Answer from the drawing. Dimensions are ordinates in mm from the lowest x, y and z of the part. A direction names the side the tool comes from. Round coordinates to 2 decimals unless told otherwise and drop trailing zeros. Write each loop counter-clockwise with the first axis right and the second up, starting at its lowest first coordinate (ties: lowest second). Pieces come first, ordered by that corner, then holes. Notation, with made-up numbers: (80, -22.5) -> (120, -22.5) arc R35 ccw to (120, 10.5) -> close; hole circle Ø2 at (-39, -21). An arc over 180 degrees is marked (long way). Return JSON: item names as keys, results as strings. Group by question number.
(1) A cutting plane is placed at B-B on x = 17. Give the vertices of the cut face in (y, z), then the cut area to 3 significant figures.
(2) A cutting plane is placed at C-C on y = 2.5. Give the vertices of the cut face in (x, z), then the cut area to 3 significant figures.
(3) A cutting plane is placed at A-A on y = 18. Give the vertices of the cut face in (x, z), then the cut area to 3 significant figures.
(4) For the marked faces 4, 5 and 6, determine the directions among +Z, -Z, +X, -X, +Y, -Y from which every point of the face is accessible in a straight line to the end or side of a thin tool.
(5) Given pin 1 (3 mm diameter, centred on y = 8.5, z = 1.5, fed in from +X); pin 2 (2 mm diameter, centred on x = 12, y = 15, fed in from -Z); pin 3 (3 mm diameter, centred on y = 17, z = 2, fed in from -X); pin 4 (2 mm diameter, centred on x = 2, z = 3.5, fed in from +Y), each flat-ended and moving along its own axis, determine where each tip first touches the part or whether it passes through.
(6) A cutting plane is placed at D-D on z = 4.9. Give the vertices of the cut face in (x, y), then the cut area to 3 significant figures.
(7) The mould has two halves that part along Z. Classify the marked faces 1, 2 and 3: released by +Z, released by -Z, zero draft, split by the parting line, or undercut.
(8) Straight lines are drawn through the part: line 1 (X direction, y = 14.5, z = 4.8); line 2 (Y direction, x = 4.65, z = 3); line 3 (X direction, y = 3.25, z = 4.1). For each, find the intervals that lie inside material, in ascending order.
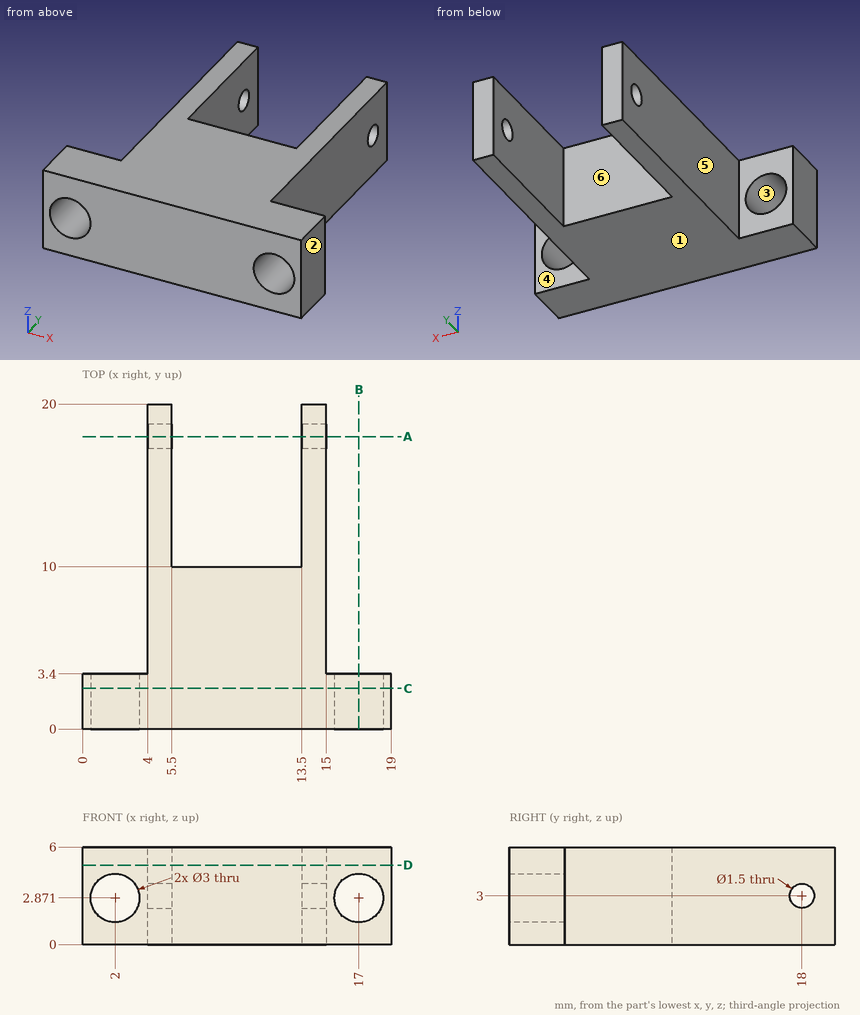
Checks:
{
 "1": {"outline": "(0, 0) -> (3.4, 0) -> (3.4, 1.37) -> (0, 1.37) -> close; (0, 4.37) -> (3.4, 4.37) -> (3.4, 6) -> (0, 6) -> close", "area": "10.2 mm^2"},
 "2": {"outline": "(0, 0) -> (19, 0) -> (19, 6) -> (0, 6) -> close; hole circle Ø3 at (2, 2.87); hole circle Ø3 at (17, 2.87)", "area": "99.9 mm^2"},
 "3": {"outline": "(4, 0) -> (5.5, 0) -> (5.5, 2.25) -> (4, 2.25) -> close; (4, 3.75) -> (5.5, 3.75) -> (5.5, 6) -> (4, 6) -> close; (13.5, 0) -> (15, 0) -> (15, 2.25) -> (13.5, 2.25) -> close; (13.5, 3.75) -> (15, 3.75) -> (15, 6) -> (13.5, 6) -> close", "area": "13.5 mm^2"},
 "4": {"face 4": "+Z, -Z, +X, +Y", "face 5": "+Z, -Z, -X, +Y", "face 6": "+Z, -Z, +Y"},
 "5": {"pin 1": "stops at x = 15", "pin 2": "passes through", "pin 3": "stops at x = 4", "pin 4": "stops at y = 3.4"},
 "6": {"outline": "(0, 0) -> (19, 0) -> (19, 3.4) -> (15, 3.4) -> (15, 20) -> (13.5, 20) -> (13.5, 10) -> (5.5, 10) -> (5.5, 20) -> (4, 20) -> (4, 3.4) -> (0, 3.4) -> close", "area": "167 mm^2"},
 "7": {"face 1": "released by -Z", "face 2": "zero draft", "face 3": "undercut"},
 "8": {"line 1": "x = 4 to 5.5, 13.5 to 15", "line 2": "y = 0 to 17.25, 18.75 to 20", "line 3": "x = 0 to 1.14, 2.86 to 16.14, 17.86 to 19"}
}
